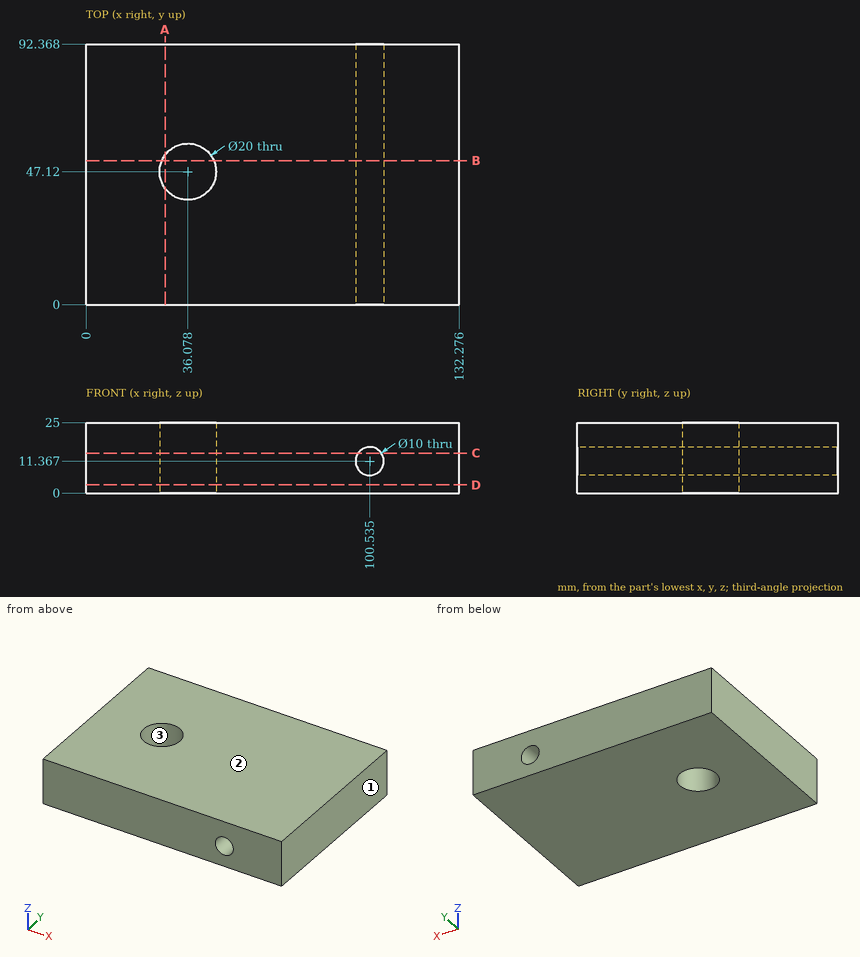
Check sheet for the drawn part. Datum: minimum x, y, z corner. Units: mm. Give positions to 0.01 mm unless a question says otherwise; leave off trailing zeros. Loops run counter-clockwise (first coordinate to the right, second up) from the corner with the lowest first, then second, coordinate; pieces in that order, holes last. Notation, with made-up numbers: (-36, 39) - (4, 39) arc R31 ccw to (4, 72) - close; hole circle Ø5 at (81.25, 81.25). An arc over 180 degrees is marked (long way). Write each question's results on one line, items separated by ' | '.
1) Sectioned sample at D-D on z = 3. Record the boundary of the cut face in (x, y), plus the area to 3 significant figures.
Solution:
outline: (0, 0) - (132.28, 0) - (132.28, 92.37) - (0, 92.37) - close; hole circle Ø20 at (36.08, 47.12) | area: 11,900 mm2
2) Mould release check, pull along X, two halves, no side actions. Record for the marked faces 1, 2 and 3: pulls with the +X half, pulls with the -X half, needs draft (parallel to the pull), parting line crosses it, or undercut.
Solution:
face 1: pulls with the +X half | face 2: needs draft | face 3: undercut
3) Sectioned sample at C-C on z = 14.25. Record the boundary of the cut face in (x, y), plus the area to 4 significant figures.
Solution:
outline: (0, 0) - (96.45, 0) - (96.45, 92.37) - (0, 92.37) - close; (104.62, 0) - (132.28, 0) - (132.28, 92.37) - (104.62, 92.37) - close; hole circle Ø20 at (36.08, 47.12) | area: 11,150 mm2
4) Sectioned sample at A-A on x = 28. Record the boundary of the cut face in (y, z) (1 decimal).
Solution:
outline: (0, 0) - (41.2, 0) - (41.2, 25) - (0, 25) - close; (53, 0) - (92.4, 0) - (92.4, 25) - (53, 25) - close
5) Material ranges on L1, parallel to X at y = 43, z = 10.25 (1 decimal); L2, parallel to Y at x = 36.5, z = 5; L3, parallel to X at y = 38, z = 21.5 (1 decimal), recorded low to high. Write a range as from..to.
Solution:
L1: 0..27, 45.2..95.7, 105.4..132.3 | L2: 0..37.13, 57.11..92.37 | L3: 0..32, 40.2..132.3
6) Sectioned sample at B-B on y = 51. Record the boundary of the cut face in (x, z) (1 decimal), plus the area to 3 significant figures.
Solution:
outline: (0, 0) - (26.9, 0) - (26.9, 25) - (0, 25) - close; (45.3, 0) - (132.3, 0) - (132.3, 25) - (45.3, 25) - close; hole circle Ø10 at (100.5, 11.4) | area: 2,770 mm2
